The figure shows three views and two pictorial views of one solid part (mm, origin at its lowest corner). Answer the questions. A direction names the side the tool comes from. Coordinates: 2 decimals unless noted, no trailing zeros. Loops run counter-clockwise (first coordinate to the right, second up) from the corner with the lowest first, then second, coordinate; pieces in that order, holes last. Notation, with made-up numbers: (-16.75, 86) - (5.25, 86) arc R15 cw to (5.25, 101) - close; hole circle Ø6 at (-14, 77). An arc over 180 degrees is marked (long way). Write each question's results on one line, items separated by ' | '. Start each with the question number.
Item 1: For a pull along X with two mould halves and no side action, classify the marked faces 3, 4 and 5 as +X half, -X half, draft (parallel to the pull), parting line (faces both ways), or undercut.
Item 2: Section A-A, the plane x = 10 is taken. Write down the section's boundary in (y, z), plus the area to 3 significant figures.
Item 3: Each of these flat-tipped pins is pushed along its axis until it touches: pin 1 Ø12 at (y, z) = (16.5, 4) entering from +X; pin 2 Ø8 at (x, z) = (8, 11) entering from +Y; pin 3 Ø12 at (y, z) = (16.5, 4) entering from -X; pin 4 Ø1 at (y, z) = (4.5, 6.5) entering from +X. Where does it stop, or does it pass through?
Item 4: Consider probe 1 along Y at (x, z) = (10, 11.75); probe 2 along X at (y, z) = (10.25, 14.5); probe 3 along Y at (x, z) = (10, 18.15). Determine where each line is inside the solid, lowest interval first. Write a range as [from, to].
Item 5: A tool of negligible diameter and unlimited length cuts with its end or side. For the marked faces 1 and 2, from which of +Z, -Z, +X, -X, +Y, -Y can it reach the whole face along a straight path? Write none if from no direction.
Item 6: Section C-C, the plane z = 4 is taken. Write down the section's boundary in (x, y), plus the area to 3 significant figures.
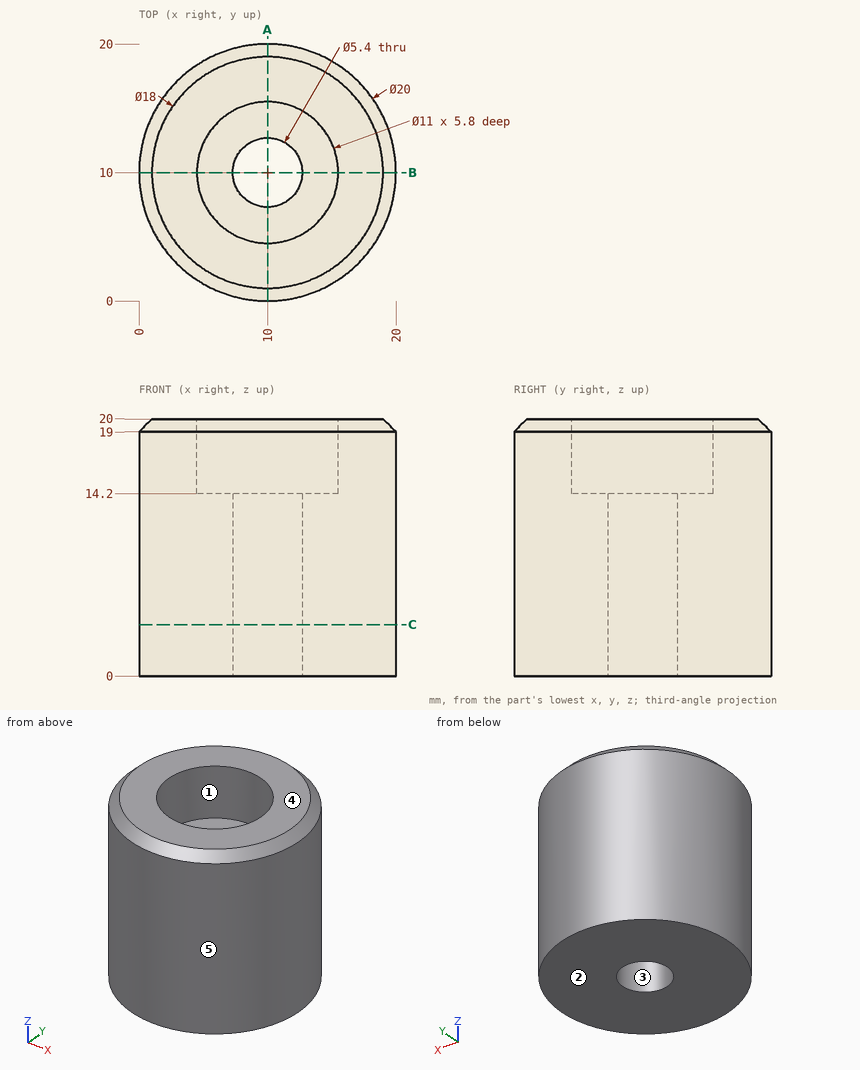
Answer key:
1) face 3: undercut | face 4: draft | face 5: parting line
2) outline: (0, 0) - (7.3, 0) - (7.3, 14.2) - (4.5, 14.2) - (4.5, 20) - (1, 20) - (0, 19) - close; (12.7, 0) - (20, 0) - (20, 19) - (19, 20) - (15.5, 20) - (15.5, 14.2) - (12.7, 14.2) - close | area: 259 mm^2
3) pin 1: stops at x = 19.99 | pin 2: stops at y = 20 | pin 3: stops at x = 0.01 | pin 4: stops at x = 18.66
4) probe 1: y = [0, 7.3], [12.7, 20] | probe 2: x = [0, 4.51], [15.49, 20] | probe 3: y = [0, 4.5], [15.5, 20]
5) face 1: +Z | face 2: -Z, +X, -X, +Y, -Y
6) outline: circle Ø20 at (10, 10); hole circle Ø5.4 at (10, 10) | area: 291 mm^2
